Read the model definition and answer for the solid it produces. Units are mm, in the model's axes. A direction names the side the tool comes from. Coordinates: 2 decimals unless noted, no trailing zeros. Write each loop counter-clockwise with the first axis right and the second up, starting at its lowest first coordinate (ties: lowest second). Pieces come first, ordered by that corner, then holes. Notation, with made-up numbers: (24, 84) -> (74, 84) arc R29 cw to (74, 110) -> close; hole circle Ø8 at (-13.5, 31). An arc over 180 degrees is marked (long way). Answer in a Markdown table with one row per item. Add a question column.
Item 1: For a pull along X with two mould halves and no side action, classify faces 3 (the face through (6.536, -0.986, 0.325)), 4 (the face through (-10.74, -0.99, 2.38)), 5 (the face through (-5, 0, -2)) as +X half, -X half, draft (parallel to the pull), parting line (faces both ways), or undercut.
Item 2: Section C-C on x = -7.25 is taken. Write down the section's boundary in (y, z), then the cut area to 3 significant figures.
Item 3: Section D-D on y = 2 is taken. Write down the section's boundary in (x, z).
Item 4: Which of the six approach directions +Z, -Z, +X, -X, +Y, -Y give full straight-line access (tool end or side, diameter ignored) to faces 1 (the face through (-6.536, -0.986, -0.325)), 2 (the face through (-2.44, 4.93, -0.54))?
Item 5: Section A-A on x = 0 is taken. Write down the section's boundary in (y, z).
Item 6: Section B-B on z = -9 is taken. Write down the section's boundary in (x, y), then the cut area to 3 significant figures.
Item 7: Given pin 1 Ø1 at (x, y) = (3.5, 1.5) entering from +Z; pin 2 Ø2.5 at (x, z) = (-1, -0.5) entering from +Y; pin 3 Ø3 at (y, z) = (0, -7) entering from -X, each flat-ended and moving along its own axis, determine where each tip first touches the part or whether it passes through.
Item 8: Straight lines are drawn through the part: line 1 (X direction, y = -1.4, z = 0); line 2 (X direction, y = 5.5, z = 0); line 3 (Z direction, x = -1, y = -0.25). For each, find the intervals that lie inside material, in ascending order. Write a range as from..to.
```python
from build123d import *

# Parameters (mm, degrees)
SKETCH_1_R      = 5
SKETCH_1_R_2    = 2.5
EXTRUDE_1_DEPTH = 10
SKETCH_2_R      = 11
SKETCH_2_R_2    = 1.5
EXTRUDE_2_DEPTH = 2


with BuildPart() as part:
    # 草图1 → 凸台-拉伸1 (new body)
    with BuildSketch(Plane(origin=(0, 0, 0), x_dir=(1, 0, 0), z_dir=(0, 1, 0))):
        with Locations(Location((0, 0, 0), (0, 0, 270))):
            Circle(SKETCH_1_R)
        with Locations(Location((0, 0, 0), (0, 0, 270))):
            Circle(SKETCH_1_R_2, mode=Mode.SUBTRACT)
    extrude(amount=EXTRUDE_1_DEPTH)

    # 草图2 → 凸台-拉伸2 (add)
    with BuildSketch(Plane.XZ):
        with Locations(Location((0, 0, 0), (0, 0, 270))):
            Circle(SKETCH_2_R)
        with Locations(Location((0, 8, 0), (0, 0, 270))):
            Circle(SKETCH_2_R_2, mode=Mode.SUBTRACT)
        with Locations(Location((8, 0, 0), (0, 0, 270))):
            Circle(SKETCH_2_R_2, mode=Mode.SUBTRACT)
        with Locations(Location((-8, 0, 0), (0, 0, 90))):
            Circle(SKETCH_2_R_2, mode=Mode.SUBTRACT)
        with Locations(Location((0, -8, 0), (0, 0, 90))):
            Circle(SKETCH_2_R_2, mode=Mode.SUBTRACT)
        with Locations(Location((0, 0, 0), (0, 0, 270))):
            Circle(SKETCH_2_R_2, mode=Mode.SUBTRACT)
    extrude(amount=EXTRUDE_2_DEPTH)


solid = part.part
```
Results below:
| question | item | result |
|---|---|---|
| 1 | face 3 | undercut |
| 1 | face 4 | parting line |
| 1 | face 5 | draft |
| 2 | outline | (-2, -8.27) -> (0, -8.27) -> (0, -1.3) -> (-2, -1.3) -> close; (-2, 1.3) -> (0, 1.3) -> (0, 8.27) -> (-2, 8.27) -> close |
| 2 | area | 27.9 mm2 |
| 3 | outline | circle Ø10 at (0, 0); hole circle Ø5 at (0, 0) |
| 4 | face 1 | +Y, -Y |
| 4 | face 2 | +Y |
| 5 | outline | (-2, -11) -> (0, -11) -> (0, -9.5) -> (-2, -9.5) -> close; (-2, -6.5) -> (0, -6.5) -> (0, -5) -> (10, -5) -> (10, -2.5) -> (0, -2.5) -> (0, -1.5) -> (-2, -1.5) -> close; (-2, 1.5) -> (0, 1.5) -> (0, 2.5) -> (10, 2.5) -> (10, 5) -> (0, 5) -> (0, 6.5) -> (-2, 6.5) -> close; (-2, 9.5) -> (0, 9.5) -> (0, 11) -> (-2, 11) -> close |
| 6 | outline | (-6.32, -2) -> (-1.12, -2) -> (-1.12, 0) -> (-6.32, 0) -> close; (1.12, -2) -> (6.32, -2) -> (6.32, 0) -> (1.12, 0) -> close |
| 6 | area | 20.8 mm2 |
| 7 | pin 1 | stops at z = 4 |
| 7 | pin 2 | stops at y = 0 |
| 7 | pin 3 | stops at x = -9.53 |
| 8 | line 1 | x = -11..-9.5, -6.5..-1.5, 1.5..6.5, 9.5..11 |
| 8 | line 2 | x = -5..-2.5, 2.5..5 |
| 8 | line 3 | z = -10.95..-9.12, -6.88..-1.12, 1.12..6.88, 9.12..10.95 |
